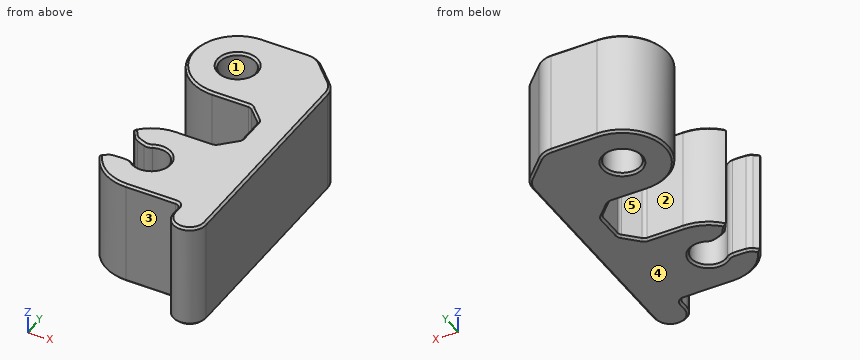
from build123d import *

# Parameters (mm, degrees)
SKETCH2_R                         = 1.575
SKETCH2_R_2                       = 1.625
BOSS_EXTRUDE1_DEPTH               = 5
LATCH_NOTCH_DEPTH                 = 21.433199089
LATCH_NOTCH_DEPTH_BACK            = 21.433199089
FILLET2_R                         = 1
THUMB_BUMP_LONG_REACH             = 22.433
THUMB_BUMP_LONG_DIRECTION_2_REACH = 22.433
FILLET6_R                         = 0.5
MOVEMENT_CLEARANCE_DEPTH          = 0.2
FILLET3_R                         = 2
FILLET4_R                         = 0.5
CHAMFER2_SIZE                     = 0.2


with BuildPart() as part:
    # Sketch2 → Boss-Extrude1 (new, symmetric)
    with BuildSketch(Plane.XY):
        with BuildLine():
            Line((8, -15.125), (8, 1.125))
            Line((8, 1.125), (5, 4.125))
            Line((5, 4.125), (0, 4.125))
            ThreePointArc((0, 4.125), (-4.125, 0), (0, -4.125))
            Line((0, -4.125), (3.5, -4.125))
            Line((3.5, -4.125), (5, -5.625))
            Line((5, -5.625), (5, -8.375))
            Line((5, -8.375), (3.5, -9.875))
            Line((3.5, -9.875), (0, -9.875))
            ThreePointArc((0, -9.875), (-4.125, -14), (0, -18.125))
            Line((0, -18.125), (5, -18.125))
            Line((5, -18.125), (8, -15.125))
        make_face()
        with Locations((0, -14)):
            Circle(SKETCH2_R, mode=Mode.SUBTRACT)
        Circle(SKETCH2_R_2, mode=Mode.SUBTRACT)
    extrude(amount=BOSS_EXTRUDE1_DEPTH, both=True)

    # Sketch3 → Latch Notch (cut, two sides: drawn at the far end of the back side and taken through both)
    with BuildSketch(Plane.XY.offset(-LATCH_NOTCH_DEPTH_BACK)):
        with BuildLine():
            Line((-5.189425986, -13.053442339), (-4.352006159, -10.311715335))
            ThreePointArc((-4.352006159, -10.311715335), (-2.519069602, -12.169061048), (0, -12.85))
            Line((0, -12.85), (0, -15.15))
            ThreePointArc((0, -15.15), (-3.063481939, -15.004958499), (-6.026845813, -15.795169343))
            Line((-6.026845813, -15.795169343), (-5.189425986, -13.053442339))
        make_face()
    extrude(amount=LATCH_NOTCH_DEPTH + LATCH_NOTCH_DEPTH_BACK, mode=Mode.SUBTRACT)

    # Chamfer1
    # the kernel refuses this chamfer: 1.535901437, 0.897551306, 0.4 mm, written as the material it takes off along each edge
    with BuildSketch(Plane(origin=(-3.336286816, -11.574136179, -7.844626154), x_dir=(0.8125376228226495, -0.5829087505756949, 0), z_dir=(0, 0, 1))) as chamfer1_piece_1:
        with BuildLine():
            Line((1.080053984, 0), (0.021291111, 0.393036797))
            ThreePointArc((0.021291111, 0.393036797), (0.006455038, 0.205821568), (0, 0))
            ThreePointArc((0, 0), (0.568931585, -0.029164914), (1.080053984, 0))
        make_face()
    extrude(amount=15.689252309, mode=Mode.SUBTRACT)
    with BuildSketch(Plane(origin=(-3.96348247, -15.142992437, -7.141629453), x_dir=(0.3226160511275448, -0.9465299168831746, 0), z_dir=(0, 0, 1))) as chamfer1_piece_2:
        with BuildLine():
            Line((0.393613053, 0), (0.141125799, 0.8123737))
            ThreePointArc((0.141125799, 0.8123737), (0.064933685, 0.423381867), (0, 0))
            ThreePointArc((0, 0), (0.202118313, -0.004694141), (0.393613053, 0))
        make_face()
    extrude(amount=14.283258906, mode=Mode.SUBTRACT)

    # Fillet2
    fillet2_edges = [part.edges().sort_by_distance(p)[0] for p in [
        (-1.235054025, -14.977377387, 0),
        (-0.965763736, -12.755843496, 0),
        (-3.149017011, -15.014487433, 0),
        (-2.45870232, -12.203709097, 0),
    ]]
    fillet(fillet2_edges, radius=FILLET2_R)

    # Thumb Bump LONG: up to this face of the body (flat: up to its plane)
    thumb_bump_long_end = Plane(part.part.faces().sort_by_distance((-2.247358014, -15.204704165, 5))[0])
    # Sketch6 → Thumb Bump LONG (add, up to the picked face)
    with BuildSketch(Plane.XY, mode=Mode.PRIVATE) as thumb_bump_long_sk1:
        with BuildLine():
            Line((8, -15.125), (8, -19.375))
            ThreePointArc((8, -19.375), (6.5, -20.875), (5, -19.375))
            Line((5, -19.375), (5, -18.125))
            Line((5, -18.125), (8, -15.125))
        make_face()
    thumb_bump_long_tool1 = split(extrude(thumb_bump_long_sk1.sketch, amount=THUMB_BUMP_LONG_REACH, mode=Mode.PRIVATE), bisect_by=thumb_bump_long_end, keep=Keep.BOTH, mode=Mode.PRIVATE)
    add(thumb_bump_long_tool1.solids().sort_by(Axis((6.690932, -18.50785, 0), (0, 0, 1)))[0])

    # Thumb Bump LONG direction 2: up to this face of the body (flat: up to its plane)
    thumb_bump_long_direction_2_end = Plane(part.part.faces().sort_by_distance((-2.247358014, -15.204704165, -5))[0])
    # Sketch6 → Thumb Bump LONG direction 2 (add, up to the picked face)
    with BuildSketch(Plane.XY, mode=Mode.PRIVATE) as thumb_bump_long_direction_2_sk1:
        with BuildLine():
            Line((8, -15.125), (8, -19.375))
            ThreePointArc((8, -19.375), (6.5, -20.875), (5, -19.375))
            Line((5, -19.375), (5, -18.125))
            Line((5, -18.125), (8, -15.125))
        make_face()
    thumb_bump_long_direction_2_tool1 = split(extrude(thumb_bump_long_direction_2_sk1.sketch, amount=-THUMB_BUMP_LONG_DIRECTION_2_REACH, mode=Mode.PRIVATE), bisect_by=thumb_bump_long_direction_2_end, keep=Keep.BOTH, mode=Mode.PRIVATE)
    add(thumb_bump_long_direction_2_tool1.solids().sort_by(Axis((6.690932, -18.50785, 0), (0, 0, -1)))[0])

    # Fillet6
    fillet6_edges = [part.edges().sort_by_distance(p)[0] for p in [
        (5, -18.125, 0),
    ]]
    fillet(fillet6_edges, radius=FILLET6_R)

    # Sketch5 → Movement Clearance (cut)
    with BuildSketch(Plane.XY.offset(5)):
        with BuildLine():
            Line((-3.367662745, -15.173848028), (-3.836496581, -15.515558967))
            ThreePointArc((-3.836496581, -15.515558967), (-2.319907785, -17.410814107), (0, -18.125))
            Line((0, -18.125), (4.5, -18.125))
            ThreePointArc((4.5, -18.125), (4.853553391, -18.271446609), (5, -18.625))
            Line((5, -18.625), (5, -19.375))
            ThreePointArc((5, -19.375), (6.5, -20.875), (8, -19.375))
            Line((8, -19.375), (8, 1.125))
            Line((8, 1.125), (5, 4.125))
            Line((5, 4.125), (0, 4.125))
            ThreePointArc((0, 4.125), (-4.125, 0), (0, -4.125))
            Line((0, -4.125), (3.5, -4.125))
            Line((3.5, -4.125), (5, -5.625))
            Line((5, -5.625), (5, -8.375))
            Line((5, -8.375), (3.5, -9.875))
            Line((3.5, -9.875), (0, -9.875))
            ThreePointArc((0, -9.875), (-1.694518043, -10.239117976), (-3.089882399, -11.267189769))
            Line((-3.089882399, -11.267189769), (-2.598457721, -11.996345718))
            ThreePointArc((-2.598457721, -11.996345718), (-2.427061693, -12.190611517), (-2.211513476, -12.334329174))
            ThreePointArc((-2.211513476, -12.334329174), (-1.819392443, -12.507232133), (-1.413905836, -12.645922256))
            ThreePointArc((-1.413905836, -12.645922256), (-1.047175867, -12.683207874), (-0.691852953, -12.585092055))
            ThreePointArc((-0.691852953, -12.585092055), (1.562261425, -14.19991058), (-1.025836674, -15.195108412))
            ThreePointArc((-1.025836674, -15.195108412), (-1.313167774, -15.022506023), (-1.641393845, -14.954547274))
            ThreePointArc((-1.641393845, -14.954547274), (-2.253812991, -14.951393788), (-2.865276684, -14.985734846))
            ThreePointArc((-2.865276684, -14.985734846), (-3.129319301, -15.04547458), (-3.367662745, -15.173848028))
        make_face()
    movement_clearance = extrude(amount=-MOVEMENT_CLEARANCE_DEPTH, mode=Mode.SUBTRACT)

    # Movement Clearance 2: Movement Clearance across plane
    add(movement_clearance.mirror(Plane.XY), mode=Mode.SUBTRACT)

    # Fillet3
    fillet3_edges = [part.edges().sort_by_distance(p)[0] for p in [
        (5, 4.125, 0),
        (8, 1.125, 0),
    ]]
    fillet(fillet3_edges, radius=FILLET3_R)

    # Fillet4
    fillet4_edges = [part.edges().sort_by_distance(p)[0] for p in [
        (3.5, -9.875, 0),
        (5, -8.375, 0),
        (5, -5.625, 0),
        (3.5, -4.125, 0),
    ]]
    fillet(fillet4_edges, radius=FILLET4_R)

    # Chamfer2
    chamfer2_edges = [part.edges().sort_by_distance(p)[0] for p in [
        (-2.319907785, -17.410814107, 4.8),
        (-3.602079663, -15.344703498, 4.8),
        (-3.129319301, -15.04547458, 4.8),
        (-2.253812991, -14.951393788, 4.8),
        (-1.313167774, -15.022506023, 4.8),
        (1.562261425, -14.19991058, 4.8),
        (-1.047175867, -12.683207874, 4.8),
        (-1.819392443, -12.507232133, 4.8),
        (-2.427061693, -12.190611517, 4.8),
        (-2.84417006, -11.631767743, 4.8),
        (-1.694518043, -10.239117976, 4.8),
        (1.646446609, -4.125, 4.8),
        (-4.125, 0, 4.8),
        (8, -9.539213562, 4.8),
        (6.5, -20.875, 4.8),
        (5, -19, 4.8),
        (4.853553391, -18.271446609, 4.8),
        (2.25, -18.125, 4.8),
        (-1.625, 0, 4.8),
        (-1.625, 0, -4.8),
        (-2.319907785, -17.410814107, -4.8),
        (2.25, -18.125, -4.8),
        (4.853553391, -18.271446609, -4.8),
        (5, -19, -4.8),
        (6.5, -20.875, -4.8),
        (8, -9.539213562, -4.8),
        (-4.125, 0, -4.8),
        (1.646446609, -4.125, -4.8),
        (-1.694518043, -10.239117976, -4.8),
        (-2.84417006, -11.631767743, -4.8),
        (-2.427061693, -12.190611517, -4.8),
        (-1.819392443, -12.507232133, -4.8),
        (-1.047175867, -12.683207874, -4.8),
        (1.562261425, -14.19991058, -4.8),
        (-1.313167774, -15.022506023, -4.8),
        (-2.253812991, -14.951393788, -4.8),
        (-3.129319301, -15.04547458, -4.8),
        (-3.602079663, -15.344703498, -4.8),
        (6.5, 2.625, -4.8),
        (6.5, 2.625, 4.8),
        (2.085786438, 4.125, -4.8),
        (4.93693974, 3.972759065, -4.8),
        (7.847759065, 1.06193974, -4.8),
        (2.085786438, 4.125, 4.8),
        (4.93693974, 3.972759065, 4.8),
        (7.847759065, 1.06193974, 4.8),
        (1.646446609, -9.875, -4.8),
        (1.646446609, -9.875, 4.8),
        (4.25, -9.125, -4.8),
        (4.25, -9.125, 4.8),
        (5, -7, -4.8),
        (5, -7, 4.8),
        (4.25, -4.875, -4.8),
        (4.25, -4.875, 4.8),
        (3.484234935, -9.836939766, -4.8),
        (3.484234935, -9.836939766, 4.8),
        (4.961939766, -8.359234935, -4.8),
        (4.961939766, -8.359234935, 4.8),
        (4.961939766, -5.640765065, -4.8),
        (4.961939766, -5.640765065, 4.8),
        (3.484234935, -4.163060234, -4.8),
        (3.484234935, -4.163060234, 4.8),
    ]]
    chamfer(chamfer2_edges, length=CHAMFER2_SIZE)


solid = part.part
Verification items for the finished model (mm, model axes). Face numbers are marked on the shaded views. A direction names the side the tool comes from. Give positions to 0.01 mm unless a question says otherwise; leave off trailing zeros. Loops run counter-clockwise (first coordinate to the right, second up) from the corner with the lowest first, then second, coordinate; pieces in that order, holes last.
1) Set-up check for the marked faces 1 and 2: record each of +Z, -Z, +X, -X, +Y, -Y from which the full face is reachable in a straight line by a thin tool's end or side.
2) Sectioned sample at B-B, the plane y = -14. Enter the section's corners in (x, z) (3 decimals), then the cut area to 3 significant figures.
3) Sectioned sample at C-C, the plane x = 6.5. Enter the section's corners in (y, z) (3 decimals), then the cut area to 3 significant figures.
4) Thickness scan on line 1 along Y through (x, z) = (0, -1.75) (3 decimals); line 2 along Y through (x, z) = (2, -3.25) (3 decimals); line 3 along X through (y, z) = (0, -0.25) (3 decimals). Record the ranges inside material, lowest first.
5) Draft check along Y on the marked faces 3, 4 and 5. Enter one of: pulls with the +Y half, pulls with the -Y half, needs draft (parallel to the pull), parting line crosses it, or undercut.
6) Sectioned sample at A-A, the plane y = 0. Enter the section's corners in (x, z) (3 decimals).
7) Depth check by flat-ended pin: pin 1 Ø1.9 at (y, z) = (-7.5, -1) entering from -X; pin 2 Ø0.6 at (y, z) = (-19, 0.5) entering from -X; pin 3 Ø1 at (x, z) = (-0.5, -3) entering from -Y (3 decimals). Enter the tip coordinate at first touch or a pass-through.
Answers:
1. face 1: +Z, -Z
1. face 2: +Z, -Z, -X
2. outline: (1.575, -4.6) - (1.775, -4.8) - (7.8, -4.8) - (8, -4.6) - (8, 4.6) - (7.8, 4.8) - (1.775, 4.8) - (1.575, 4.6) - close
2. area: 61.6 mm2
3. outline: (-20.875, -4.6) - (-20.675, -4.8) - (2.342, -4.8) - (2.625, -4.6) - (2.625, 4.6) - (2.342, 4.8) - (-20.675, 4.8) - (-20.875, 4.6) - close
3. area: 226 mm2
4. line 1: y = -18.125 to -15.575, -12.425 to -9.875, -4.125 to -1.625, 1.625 to 4.125
4. line 2: y = -18.125 to -9.875, -4.125 to 4.125
4. line 3: x = -4.125 to -1.625, 1.625 to 8
5. face 3: pulls with the -Y half
5. face 4: needs draft
5. face 5: undercut
6. outline: (-4.125, -4.6) - (-3.925, -4.8) - (-1.825, -4.8) - (-1.625, -4.6) - (-1.625, 4.6) - (-1.825, 4.8) - (-3.925, 4.8) - (-4.125, 4.6) - close; (1.625, -4.6) - (1.825, -4.8) - (7.8, -4.8) - (8, -4.6) - (8, 4.6) - (7.8, 4.8) - (1.825, 4.8) - (1.625, 4.6) - close
7. pin 1: stops at x = 4.91
7. pin 2: stops at x = 5
7. pin 3: stops at y = -18.125
